Input: part model. Units: mm. Frame: model coordinates. A direction names the side the tool comes from. Give positions to 0.01 mm unless a question says otherwise; leave off trailing zeros. Write each loop counter-clockwise with the first axis right and the second up, starting at its lowest first coordinate (ties: lowest second). Pieces come first, ordered by that corner, then holes. Notation, with made-up numbers: (36.25, 82.25) -> (69.25, 82.25) arc R17 ccw to (69.25, 89.25) -> close; hole circle Ø8 at (-2, -32). An arc over 180 degrees is marked (long way). Answer as a JSON object with one key per item and string values. Group by question number.
from build123d import *

# Parameters (mm, degrees)
BOSS_EXTRUDE1_DEPTH = 4
BOSS_EXTRUDE1_DRAFT = 1
SHELL1_T            = -0.5
SKETCH2_R           = 2
BOSS_EXTRUDE2_DEPTH = 5.5
BOSS_EXTRUDE2_TAPER = 1.5
CIRPATTERN1_COUNT   = 4


with BuildPart() as part:
    # Sketch1 → Boss-Extrude1 (with draft: the straight prism first)
    with BuildSketch(Plane(origin=(0, 0, 0), x_dir=(1, 0, 0), z_dir=(0, 1, 0))):
        with BuildLine():
            Line((-7.5, -4), (7.5, -4))
            ThreePointArc((7.5, -4), (8.207106781, -3.707106781), (8.5, -3))
            Line((8.5, -3), (8.5, 3))
            ThreePointArc((8.5, 3), (8.207106781, 3.707106781), (7.5, 4))
            Line((7.5, 4), (-7.5, 4))
            ThreePointArc((-7.5, 4), (-8.207106781, 3.707106781), (-8.5, 3))
            Line((-8.5, 3), (-8.5, -3))
            ThreePointArc((-8.5, -3), (-8.207106781, -3.707106781), (-7.5, -4))
        make_face()
    extrude(amount=-BOSS_EXTRUDE1_DEPTH)
    # Boss-Extrude1: the draft: its side faces are tilted about the plane it starts from
    boss_extrude1_sides = [part.faces().sort_by_distance(p)[0] for p in [
        (0, -2, 4),
        (8.207106781, -2, 3.707106781),
        (8.5, -2, 0),
        (8.207106781, -2, -3.707106781),
        (0, -2, -4),
        (-8.207106781, -2, -3.707106781),
        (-8.5, -2, 0),
        (-8.207106781, -2, 3.707106781),
    ]]
    draft(boss_extrude1_sides, Plane(origin=(0, 0, 0), x_dir=(1, 0, 0), z_dir=(0, 1, 0)), BOSS_EXTRUDE1_DRAFT)

    # Shell1
    shell1_openings = [part.faces().sort_by_distance(p)[0] for p in [
        (0, -4, 0),
    ]]
    offset(amount=SHELL1_T, openings=shell1_openings, kind=Kind.INTERSECTION)

    # Sketch2 → Boss-Extrude2 (add)
    with BuildSketch(Plane.XZ.offset(0.5)):
        Circle(SKETCH2_R)
    extrude(amount=BOSS_EXTRUDE2_DEPTH, taper=BOSS_EXTRUDE2_TAPER)

    # Rib1: read off the stored shape, not the designer's step
    # Rib1: loft between two sections, ruled curve by curve
    rib1_from = [
        Edge.make_line((1.982021306, -0.5, 0.267565961), (3, -0.5, 0.25)),
        Edge.make_line((1.982021306, -0.5, -0.267565961), (3, -0.5, -0.25)),
        Edge.make_line((3, -0.5, -0.25), (3, -0.5, 0.25)),
        Edge.make_line((1.982021306, -0.5, -0.267565961), (1.982021306, -0.5, 0.267565961)),
    ]
    rib1_to = [
        Edge.make_line((1.877496814, -4.5, 0.25884785), (2.390245469, -4.5, 0.25)),
        Edge.make_line((1.877496814, -4.5, -0.25884785), (2.390245469, -4.5, -0.25)),
        Edge.make_line((2.390245469, -4.5, -0.25), (2.390245469, -4.5, 0.25)),
        Edge.make_line((1.877496814, -4.5, -0.25884785), (1.877496814, -4.5, 0.25884785)),
    ]
    rib1 = Solid(Shell([*[Face.make_surface_from_curves(rib1_from[k], rib1_to[k]) for k in range(4)], Face(Wire(rib1_from)), Face(Wire(rib1_to))]))
    add(rib1)

    # CirPattern1: Rib1 ×4 about axis
    cirpattern1_axis = Axis((0, 0, 0), (0, 1, 0))
    for i in range(1, CIRPATTERN1_COUNT):
        add(rib1.rotate(cirpattern1_axis, i * 360 / CIRPATTERN1_COUNT))


solid = part.part
1. Line query: line 1 (Z direction, x = 4, y = -3.75); line 2 (X direction, y = -0.75, z = -0.75); line 3 (Z direction, x = -1.5, y = -2). Output: solid intervals per line, ascending.
2. Section B-B (y = -3.25). State how many separate pieces and enclosed holes the cut face has, plus the area to 3 significant figures.
3. Section A-A (x = -3.5). Return the cut outline in (y, z), plus the area to 3 significant figures.
4. Section D-D (y = -5.25). Return the cut outline in (x, z).
5. Mould query, pull axis Z, two halves, no side actions, for faces 1 (the face through (-8.24, -1.97, 3.72)), 2 (the face through (-8.22, -1.97, -3.74)), 3 (the face through (-2, -0.5, -1)), 4 (the face through (0, -4, 3.9)). Classes: pulls with the +Z half, pulls with the -Z half, needs draft (parallel to the pull), parting line crosses it, or undercut.
6. Contact query for flat-ended pins moving along their axis: pin 1 Ø3.5 at (x, z) = (-3, -1) entering from -Y; pin 2 Ø3 at (y, z) = (-2, -3) entering from -X. Output: stop coordinate, or through.
7. Reachability of faces 5 (the face through (8.22, -1.97, 3.74)), 6 (the face through (0.89, -3.29, -1.71)), 7 (the face through (8.24, -1.97, -3.72)), 8 (the face through (0, 0, 0)) from +Z, -Z, +X, -X, +Y, -Y: full face, straight path, thin tool, end or side. Return the list, or none.
Working result:
{
 "1": {"line 1": "z = -4.07 to -3.57, 3.57 to 4.07", "line 2": "x = -8.51 to -8.01, -1.85 to 1.85, 8.01 to 8.51", "line 3": "z = -4.03 to -3.53, -1.26 to 1.26, 3.53 to 4.03"},
 "2": {"separate pieces": "2", "enclosed holes": "1", "area": "36.6 mm^2"},
 "3": {"outline": "(-4, -4.07) -> (0, -4) -> (0, 4) -> (-4, 4.07) -> (-4, 3.57) -> (-0.5, 3.51) -> (-0.5, -3.51) -> (-4, -3.57) -> close", "area": "7.50 mm^2"},
 "4": {"outline": "circle Ø3.75 at (0, 0)"},
 "5": {"face 1": "pulls with the +Z half", "face 2": "pulls with the -Z half", "face 3": "undercut", "face 4": "needs draft"},
 "6": {"pin 1": "stops at y = -6", "pin 2": "stops at x = -8.56"},
 "7": {"face 5": "+Z, +X, +Y", "face 6": "-Y", "face 7": "-Z, +X, +Y", "face 8": "+Z, -Z, +X, -X, +Y"}
}
